Design review of the part built by this model. Coordinates are the model's own, in mm. Face numbers are marked on the shaded views. A direction names the side the tool comes from. Give positions to 0.01 mm unless a question says otherwise; leave off trailing zeros. Loops run counter-clockwise (first coordinate to the right, second up) from the corner with the lowest first, then second, coordinate; pieces in that order, holes last. Notation, with made-up numbers: (13, 47) - (43, 47) arc R11 ccw to (43, 64) - close; hole circle Ø10 at (48.25, 22.5). An arc over 180 degrees is marked (long way). One line per item, written item: value. Start each with the question number.
```python
from build123d import *

# Parameters (mm, degrees)
F0_W     = 36
F0_H     = 98
F1_DEPTH = 550
F3_DEPTH = 36
F5_DEPTH = 18


with BuildPart() as f1:
    # F0 (on Front) → F1 (new body)
    with BuildSketch(Plane.XZ):
        Rectangle(F0_W, F0_H)
    extrude(amount=F1_DEPTH)

    # F2 (on face) → F3 (cut, through all)
    with BuildSketch(Plane.YZ.offset(18)):
        Polygon((-523.740979, -49), (-550, 49), (-550, -49), align=None)
    extrude(amount=-F3_DEPTH, mode=Mode.SUBTRACT)

    # F4 (on face) → F5 (cut)
    with BuildSketch(Plane.YZ.offset(18)):
        Polygon((-479.5, 49), (-550, 49), (-523.740979, -49), (-453.240979, -49), align=None)
    extrude(amount=-F5_DEPTH, mode=Mode.SUBTRACT)


solid = f1.part
```
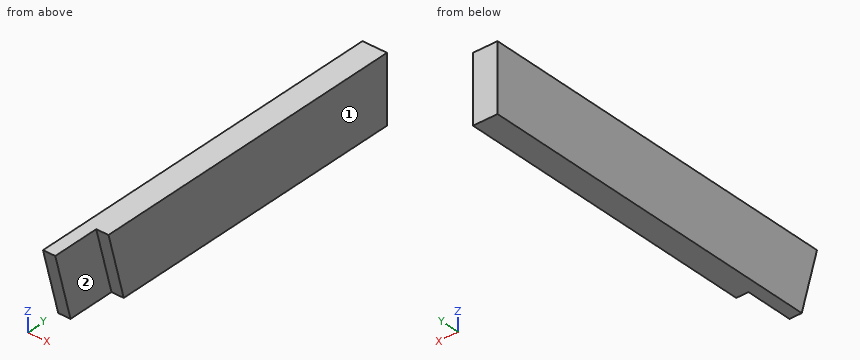
(1) Machinability: for the marked faces 1 and 2, which of the approach directions +Z, -Z, +X, -X, +Y, -Y give a long, thin tool a straight path to every point of the face, cutting with its end or side? Answer none if there is none.
(2) Take a section at A-A on x = 7.5. State the section outline as (y, z) points.
(3) To check wall thickness, follow L1, parallel to X at y = -505, z = 37; L2, parallel to Y at x = 12.5, z = 14; L3, parallel to Y at x = 15.5, z = -17.5. State the ranges of each line that lie inside material, in increasing order. Write a range as from..to.
(4) Take a section at C-C on y = -469.5. State the section outline as (x, z) points, and give its area (3 significant figures).
(5) Take a section at B-B on z = -33.5. State the section outline as (x, y) points, and give its area (3 significant figures).
(6) For pin 1 Ø5 at (x, z) = (12, 25.5) entering from +Y; pin 2 Ø1.5 at (x, z) = (12, 18.5) entering from -Y; pin 3 Ø12 at (x, z) = (-3, 30.5) entering from -Y, all flat-tipped, find the tip position at first contact; note any pin that passes through.
Here are the results:
1. face 1: +Z, -Z, +X, +Y, -Y
1. face 2: -Z, +X, -Y
2. outline: (-479.5, 49) - (-453.24, -49) - (0, -49) - (0, 49) - close
3. L1: -18..0
3. L2: -470.12..0
3. L3: -461.68..0
4. outline: (-18, -49) - (0, -49) - (0, 11.68) - (18, 11.68) - (18, 49) - (-18, 49) - close
4. area: 2,440 mm²
5. outline: (-18, -527.89) - (0, -527.89) - (0, -457.39) - (18, -457.39) - (18, 0) - (-18, 0) - close
5. area: 17,700 mm²
6. pin 1: y = 0
6. pin 2: y = -471.53
6. pin 3: y = -546.65
